Geometry check sheet. Reference: drawing and pictorial views, mm from the part's lowest x, y, z. Round coordinates to 2 decimals unless told otherwise and drop trailing zeros. Order: outer loops, then holes, each group sorted by start corner. A loop starts at its lowest first (then second) coordinate and runs counter-clockwise, first axis right, second up.
(1) Cross-section at A-A on y = 25. Enter the section's corners in (x, z) (1 decimal), and give its area (3 significant figures).
(2) Draft check along Y on the marked faces 1, 2 and 3. Enter one of: pulls with the +Y half, pulls with the -Y half, needs draft (parallel to the pull), parting line crosses it, or undercut.
(3) Cross-section at B-B on x = 50. Enter the section's corners in (y, z) (1 decimal).
(4) Cross-section at D-D on y = 44. Enter the section's corners in (x, z) (1 decimal), and give its area (3 significant figures).
(5) Cross-section at C-C on z = 22. Enter the section's corners in (x, y) (1 decimal).
(6) Thickness scan on L1, parallel to Y at x = 73, z = 29.5; L2, parallel to X at y = 25, z = 34 (1 decimal); L3, parallel to X at y = 17.5, z = 21.5 (1 decimal). Record the ranges inside material, lowest first.
(7) Gauge pin test, flat ends, axial feed: P1, Ø5, axis at y = 22, z = 44, coming from the -X side; P2, Ø3, axis at y = 34, z = 42.5, coming from the -X side (1 decimal); P3, Ø1, axis at y = 8.5, z = 8, coming from the -X side (1 decimal). Record the tip position at first contact, or that the pin passes through.
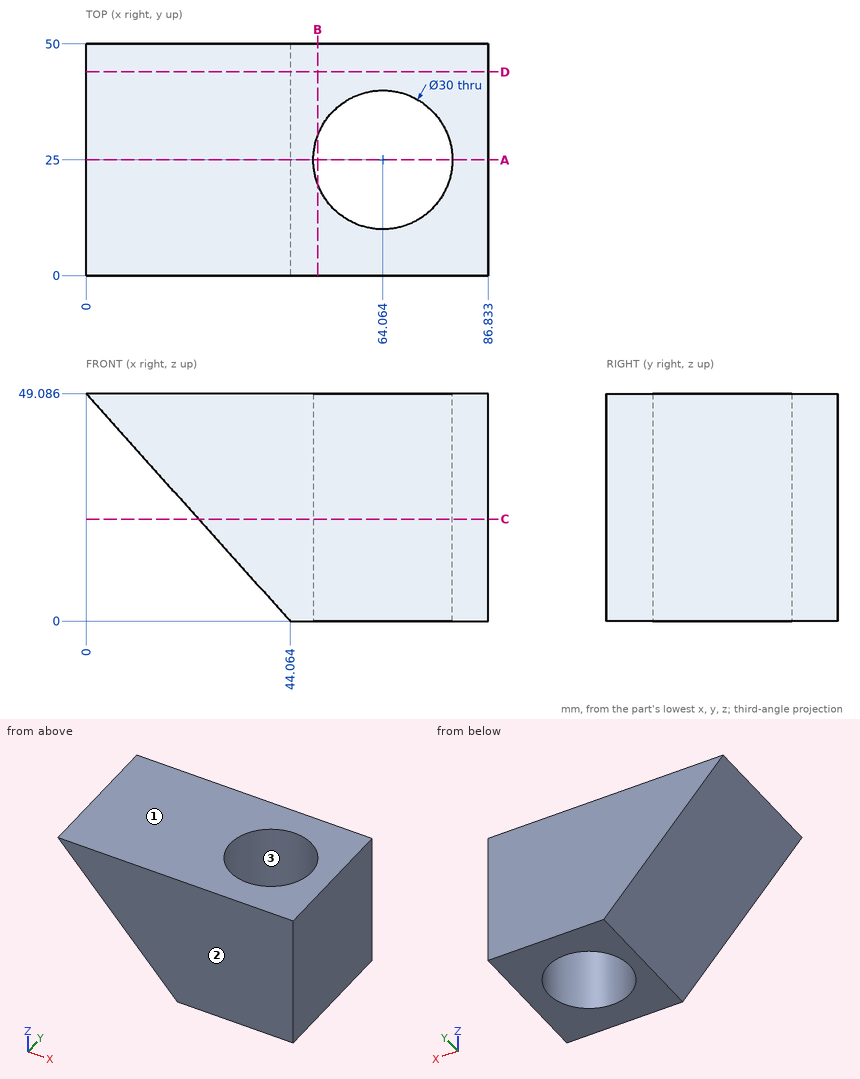
Found:
1. outline: (0, 49.1) - (44.1, 0) - (49.1, 0) - (49.1, 49.1) - close; (79.1, 0) - (86.8, 0) - (86.8, 49.1) - (79.1, 49.1) - close
1. area: 1,710 mm2
2. face 1: needs draft
2. face 2: pulls with the -Y half
2. face 3: undercut
3. outline: (0, 0) - (19.8, 0) - (19.8, 49.1) - (0, 49.1) - close; (30.2, 0) - (50, 0) - (50, 49.1) - (30.2, 49.1) - close
4. outline: (0, 49.1) - (44.1, 0) - (86.8, 0) - (86.8, 49.1) - close
4. area: 3,180 mm2
5. outline: (24.3, 0) - (86.8, 0) - (86.8, 50) - (24.3, 50) - close; hole circle Ø30 at (64.1, 25)
6. L1: y = 0 to 12.95, 37.05 to 50
6. L2: x = 13.5 to 49.1, 79.1 to 86.8
6. L3: x = 24.8 to 51.1, 77.1 to 86.8
7. P1: stops at x = 2.32
7. P2: stops at x = 4.6
7. P3: stops at x = 36.4
